Check sheet for the modelled part. Datum: model origin and axes. Units: mm. Face numbers are marked on the shaded views. A direction names the side the tool comes from. Coordinates: 2 decimals unless noted, no trailing zeros. Loops run counter-clockwise (first coordinate to the right, second up) from the corner with the lowest first, then second, coordinate; pieces in that order, holes last. Notation, with made-up numbers: M -1.75,71 L 10.25,71 A25 cw 10.25,87 Z; hole C 5,5 d9. An arc over 180 degrees is marked long. Return JSON: item names as keys, results as strings.
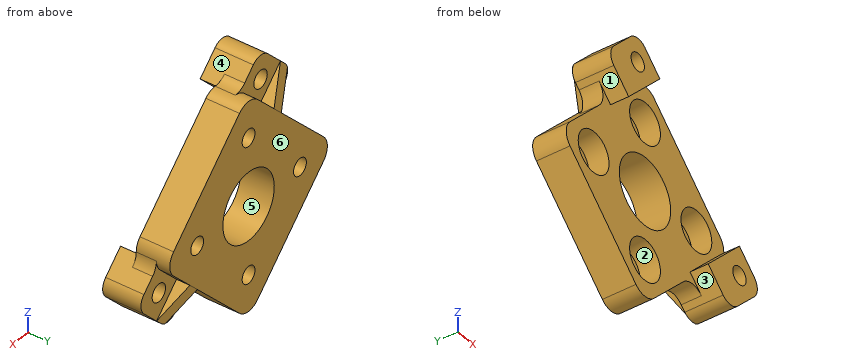
from build123d import *

# Parameters (mm, degrees)
SKETCH1_R           = 1.25
SKETCH1_R_2         = 5
BOSS_EXTRUDE1_DEPTH = 5
SKETCH4_R           = 3
CUT_EXTRUDE2_DEPTH  = 3
SKETCH3_R           = 1.3
BOSS_EXTRUDE4_DEPTH = 5.7
BOSS_EXTRUDE6_DEPTH = 1
FILLET1_R           = 2.5
FILLET2_R           = 2


with BuildPart() as part:
    # Sketch1 → Boss-Extrude1 (new body)
    with BuildSketch(Plane(origin=(0, 0, 0), x_dir=(1, 0, 0), z_dir=(0, 1, 0))):
        with BuildLine():
            Line((1.767766953, 14.596194078), (14.596194078, 1.767766953))
            ThreePointArc((14.596194078, 1.767766953), (15.328427125, 0), (14.596194078, -1.767766953))
            Line((14.596194078, -1.767766953), (1.767766953, -14.596194078))
            ThreePointArc((1.767766953, -14.596194078), (0, -15.328427125), (-1.767766953, -14.596194078))
            Line((-1.767766953, -14.596194078), (-14.596194078, -1.767766953))
            ThreePointArc((-14.596194078, -1.767766953), (-15.328427125, 0), (-14.596194078, 1.767766953))
            Line((-14.596194078, 1.767766953), (-1.767766953, 14.596194078))
            ThreePointArc((-1.767766953, 14.596194078), (0, 15.328427125), (1.767766953, 14.596194078))
        make_face()
        with Locations(Location((0, 10, 0), (0, 0, 270))):
            Circle(SKETCH1_R, mode=Mode.SUBTRACT)
        with Locations(Location((0, -10, 0), (0, 0, 270))):
            Circle(SKETCH1_R, mode=Mode.SUBTRACT)
        with Locations(Location((10, 0, 0), (0, 0, 270))):
            Circle(SKETCH1_R, mode=Mode.SUBTRACT)
        with Locations(Location((-10, 0, 0), (0, 0, 270))):
            Circle(SKETCH1_R, mode=Mode.SUBTRACT)
        with Locations(Location((0, 0, 0), (0, 0, 270))):
            Circle(SKETCH1_R_2, mode=Mode.SUBTRACT)
    extrude(amount=BOSS_EXTRUDE1_DEPTH)

    # Sketch4 → Cut-Extrude2 (cut)
    with BuildSketch(Plane.XZ):
        with Locations(Location((0, 10, 0), (0, 0, 270))):
            Circle(SKETCH4_R)
        with Locations(Location((10, 0, 0), (0, 0, 270))):
            Circle(SKETCH4_R)
        with Locations(Location((-10, 0, 0), (0, 0, 270))):
            Circle(SKETCH4_R)
        with Locations(Location((0, -10, 0), (0, 0, 270))):
            Circle(SKETCH4_R)
    extrude(amount=-CUT_EXTRUDE2_DEPTH, mode=Mode.SUBTRACT)

    # Sketch3 → Boss-Extrude4 (add)
    # profile 1 of 4: a face of its own
    with BuildSketch(Plane(origin=(0, -2.7, 0), x_dir=(1, 0, 0), z_dir=(0, 1, 0))):
        Polygon((-4.949747468, -10.537489101), (-0.637994164, -14.849242405), (-4.949747468, -19.160995709), (-9.261500772, -14.849242405), align=None)
        with Locations(Location((-4.949747468, -14.849242405, 0), (0, 0, 90))):
            Circle(SKETCH3_R, mode=Mode.SUBTRACT)
    # profile 2 of 4: a face of its own
    with BuildSketch(Plane(origin=(0, -2.7, 0), x_dir=(1, 0, 0), z_dir=(0, 1, 0))):
        Polygon((-6.717514421, -8.769722148), (-11.029267725, -13.081475452), (-9.261500772, -14.849242405), (-4.949747468, -10.537489101), align=None)
    # profile 3 of 4: a face of its own
    with BuildSketch(Plane(origin=(0, -2.7, 0), x_dir=(1, 0, 0), z_dir=(0, 1, 0))):
        Polygon((19.160995709, 4.949747468), (14.849242405, 9.261500772), (10.537489101, 4.949747468), (14.849242405, 0.637994164), align=None)
        with Locations(Location((14.849242405, 4.949747468, 0), (0, 0, 90))):
            Circle(SKETCH3_R, mode=Mode.SUBTRACT)
    # profile 4 of 4: a face of its own
    with BuildSketch(Plane(origin=(0, -2.7, 0), x_dir=(1, 0, 0), z_dir=(0, 1, 0))):
        Polygon((13.081475452, 11.029267725), (14.849242405, 9.261500772), (10.537489101, 4.949747468), (8.769722148, 6.717514421), align=None)
    extrude(amount=BOSS_EXTRUDE4_DEPTH)


with BuildPart() as boss_extrude6_tool:
    # Sketch7 → Boss-Extrude6 (new, symmetric)
    with BuildSketch(Plane(origin=(2.525126055, -2.13e-07, 2.525126055), x_dir=(0.7071067811865474, 0, -0.7071067811865477), z_dir=(0.7071067811865465, -5.960464483662305e-08, 0.7071067811865461))):
        Polygon((11.571067812, 5.000000541), (17.04887, 3.000000599), (11.571067812, 3.000000541), align=None)
        Polygon((-11.571067812, 5.000000541), (-17.04887, 3.000000599), (-11.571067812, 3.000000541), align=None)
    extrude(amount=BOSS_EXTRUDE6_DEPTH, both=True)


with BuildPart() as part_1:
    add(part.part)


with BuildPart() as part_2:
    # Boss-Extrude6: joined with boss_extrude6_tool
    add(part_1.part.fuse(boss_extrude6_tool.part, tol=0.00001))

    # Fillet1
    fillet1_edges = [part_2.edges().sort_by_distance(p)[0] for p in [
        (-7.155876652, 1.5, 9.208084379),
        (-0.935534875, 1.5, 15.146783115),
        (9.208084379, 1.5, -7.155876652),
        (15.146783115, 1.5, -0.935534875),
    ]]
    fillet(fillet1_edges, radius=FILLET1_R)

    # Fillet2
    # the kernel refuses this fillet: 2 mm, written as the material it takes off along each edge
    with BuildSketch(Plane(origin=(-4.949747468, -7.7, 19.160995709), x_dir=(-0.7071067811865471, 0, -0.707106781186548), z_dir=(0, 1, 0)), Plane(origin=(13.081475452, -7.7, -11.029267725), x_dir=(0.7071067811865476, 0, 0.7071067811865476), z_dir=(0, 1, 0))) as fillet2_piece_1:
        with BuildLine():
            CenterArc((FILLET2_R, -FILLET2_R), FILLET2_R, 90, 90)
            Line((0, -FILLET2_R), (0, 0))
            Line((0, 0), (FILLET2_R, 0))
        make_face()
    extrude(amount=15.7, mode=Mode.SUBTRACT)
    with BuildSketch(Plane(origin=(-11.029267725, -7.7, 13.081475452), x_dir=(0.707106781186547, 0, 0.7071067811865479), z_dir=(0, 1, 0)), Plane(origin=(19.160995709, -7.7, -4.949747468), x_dir=(-0.7071067811865482, 0, -0.7071067811865469), z_dir=(0, 1, 0))) as fillet2_piece_2:
        with BuildLine():
            CenterArc((FILLET2_R, FILLET2_R), FILLET2_R, 180, 90)
            Line((0, FILLET2_R), (0, 0))
            Line((0, 0), (FILLET2_R, 0))
        make_face()
    extrude(amount=15.7, mode=Mode.SUBTRACT)


solid = part_2.part
1) Section check D-D on y = 2. Count the separate pieces of the cut face and the enclosed holes in it, then the cut area to 3 significant figures.
Answers:
{"separate pieces": "1", "enclosed holes": "7", "area": "422 mm²"}
2) Section check C-C on z = 3.5. Record the cut outline in (x, y), then the cut area to 3 significant figures.
Answers:
{"outline": "M -12.86,0 L -3.57,0 L -3.57,5 L -12.86,5 Z; M 3.57,0 L 12.86,0 L 12.86,5 L 3.57,5 Z", "area": "92.9 mm²"}
3) Section check A-A on y = -0.5. Record the cut outline in (x, z), then the cut area to 3 significant figures.
Answers:
{"outline": "M -9.62,11.67 L -6.72,8.77 L -0.64,14.85 L -3.54,17.75 A2 ccw -6.36,17.75 L -9.62,14.5 A2 ccw Z; M 8.77,-6.72 L 11.67,-9.62 A2 ccw 14.5,-9.62 L 17.75,-6.36 A2 ccw 17.75,-3.54 L 14.85,-0.64 Z; hole C -4.95,14.85 d2.6; hole C 14.85,-4.95 d2.6", "area": "90.8 mm²"}
4) Scan lines: line 1 along X through (y, z) = (1.75, 0); line 2 along X through (y, z) = (3.55, 0); line 3 along Y through (x, z) = (5.5, 10). Record each from-to range of solid material in increasing order. Write a range as [from, to].
Answers:
{"line 1": "[-15.33, -13], [-7, -5], [5, 7], [13, 15.33]", "line 2": "[-15.33, -11.25], [-8.75, -5], [5, 8.75], [11.25, 15.33]", "line 3": "[0, 5]"}
5) Go/stop test with flat-tipped pins: pin 1 Ø3.5 at (x, z) = (10, 0) entering from -Y; pin 2 Ø1.9 at (x, z) = (-7.5, 10.5) entering from +Y; pin 3 Ø3 at (x, z) = (-8.5, -1) entering from -Y. Record where each tip stops, or that it passes through.
Answers:
{"pin 1": "y = 3", "pin 2": "y = 4.88", "pin 3": "y = 0"}
6) Draft check along Z on the marked faces 4, 5 and 6. Enter one of: +Z half, -Z half, draft (parallel to the pull), parting line (faces both ways), or undercut.
Answers:
{"face 4": "+Z half", "face 5": "undercut", "face 6": "draft"}
7) Section check B-B on x = -4.5. Record the cut outline in (y, z).
Answers:
{"outline": "M -2.7,10.99 L 0,10.99 L 0,2.18 L 5,2.18 L 5,11.86 L 3,11.86 L 3,13.63 L -2.7,13.63 Z; M -2.7,16.07 L 3,16.07 L 3,18.28 L -2.7,18.28 Z; M 0,-11.86 L 5,-11.86 L 5,-2.18 L 0,-2.18 Z"}
8) Set-up check for the marked faces 1, 2 and 3: record each of +Z, -Z, +X, -X, +Y, -Y from which the full face is reachable in a straight line by a thin tool's end or side.
Answers:
{"face 1": "-X, -Y", "face 2": "-Y", "face 3": "-Z, -Y"}
